Geometry check sheet. Reference: the model listing, model coordinates, mm. Face numbers are marked on the shaded views. Coordinates: 2 decimals unless noted, no trailing zeros. Order: outer loops, then holes, each group sorted by start corner. A loop starts at its lowest first (then second) coordinate and runs counter-clockwise, first axis right, second up. Notation, with made-up numbers: M -18,54 L 6,54 A14 cw 6,69 Z; hole C -9,37.25 d9. An arc over 180 degrees is marked long. One line per item, written item: value. Start each with the question number.
1) Sectioned sample at D-D, the plane y = 141.5. Enter the section's corners in (x, z).
2) Go/stop test with flat-tipped pins: P1, Ø6, axis at x = -0.5, y = -138.5, coming from the +Z side; P2, Ø6, axis at x = 136, z = -135.5, coming from the +Y side; P3, Ø1.5, axis at x = -3, z = -136.5, coming from the +Y side. Record where each tip stops, or that it passes through.
3) Sectioned sample at B-B, the plane y = 105.5. Enter the section's corners in (x, z), then the cut area to 3 significant figures.
4) Thickness scan on L1, parallel to Y at x = 0, z = 1; L2, parallel to X at y = 0, z = -6. Record the ranges inside material, lowest first. Write a range as from..to.
5) Draft check along X on the marked faces 1, 2, 3 and 4. Enter one of: pulls with the +X half, pulls with the -X half, needs draft (parallel to the pull), parting line crosses it, or undercut.
6) Sectioned sample at C-C, the plane z = -127. Enter the section's corners in (x, y) (3 decimals).
7) Sectioned sample at A-A, the plane x = 89. Enter the section's corners in (y, z), then the cut area to 3 significant figures.
```python
from build123d import *

# Parameters (mm, degrees)
F0_R        = 170
F0_R_2      = 128.5
F1_DEPTH    = 7.5
F1_FACE_R   = 170
F1_FACE_R_2 = 128.5
F2_DEPTH    = 12.5
F3_R        = 15
F4_DEPTH    = 150
F5_R        = 10
F6_DEPTH    = 8
F7_DEPTH    = 9
F8_W        = 515.232772
F8_H        = 2.5


with BuildPart() as f1:
    # F0 (on Top) → F1 (new body)
    with BuildSketch(Plane.XY):
        Circle(F0_R)
        Circle(F0_R_2, mode=Mode.SUBTRACT)
    extrude(amount=F1_DEPTH)

    # F1_face (on face) → F2 (join)
    with BuildSketch(Plane(origin=(0, 0, 0), x_dir=(1, 0, 0), z_dir=(0, 0, -1))):
        Circle(F1_FACE_R)
        Circle(F1_FACE_R_2, mode=Mode.SUBTRACT)
    extrude(amount=F2_DEPTH)

    # F3 (on face) → F4 (join)
    with BuildSketch(Plane(origin=(0, 0, -12.5), x_dir=(1, 0, 0), z_dir=(0, 0, -1))):
        with Locations((0, 149.25)):
            Circle(F3_R)
        with Locations((129.254292, -74.625)):
            Circle(F3_R)
        with Locations((-129.254292, -74.625)):
            Circle(F3_R)
    extrude(amount=F4_DEPTH)

    # F5 (on face) → F6 (cut)
    with BuildSketch(Plane.XY.offset(7.5)):
        with Locations((0, 141.5)):
            Circle(F5_R)
    extrude(amount=-F6_DEPTH, mode=Mode.SUBTRACT)

    # F5 (on face) → F7 (cut)
    with BuildSketch(Plane.XY.offset(7.5)):
        with Locations((0, -141.5)):
            Circle(F5_R)
    extrude(amount=-F7_DEPTH, mode=Mode.SUBTRACT)

    # F8 (on Top) → F9 (revolve, cut)
    with BuildSketch(Plane.XY):
        with Locations((21.541521, 1.25)):
            Rectangle(F8_W, F8_H)
    revolve(axis=Axis((21.541521, 0, 0), (1, 0, 0)), mode=Mode.SUBTRACT)


solid = f1.part
```
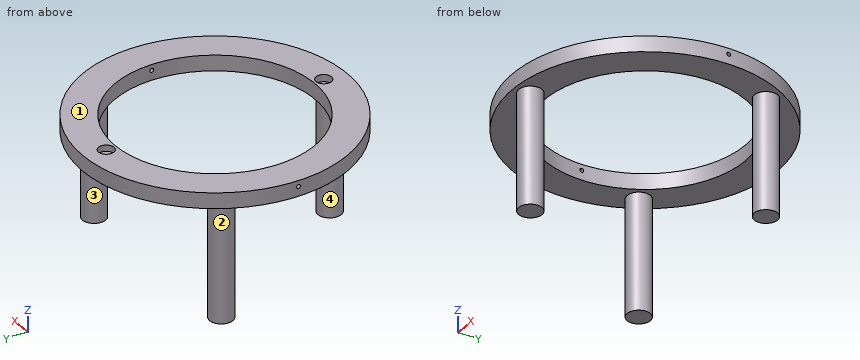
Final values:
1. outline: M -94.22,-12.5 L 94.22,-12.5 L 94.22,7.5 L 10,7.5 L 10,-0.5 L -10,-0.5 L -10,7.5 L -94.22,7.5 Z
2. P1: stops at z = -1.5
2. P2: stops at y = 89.15
2. P3: stops at y = -134.42
3. outline: M -133.3,-12.5 L -73.36,-12.5 L -73.36,7.5 L -133.3,7.5 Z; M 73.36,-12.5 L 133.3,-12.5 L 133.3,7.5 L 73.36,7.5 Z
3. area: 2,400 mm^2
4. L1: y = -170..-151.5, -131.5..-128.5, 128.5..131.5, 151.5..170
4. L2: x = -170..-128.5, 128.5..170
5. face 1: needs draft
5. face 2: undercut
5. face 3: undercut
5. face 4: parting line crosses it
6. outline: C -129.254,74.625 d30; C 0,-149.25 d30; C 129.254,74.625 d30
7. outline: M -144.84,-12.5 L -92.69,-12.5 L -92.69,7.5 L -144.84,7.5 Z; M 92.69,-12.5 L 144.84,-12.5 L 144.84,7.5 L 92.69,7.5 Z
7. area: 2,090 mm^2
